Check sheet for the modelled part. Datum: model origin and axes. Units: mm. Coordinates: 2 decimals unless noted, no trailing zeros. Order: outer loops, then holes, each group sorted by start corner. A loop starts at its lowest first (then second) coordinate and runs counter-clockwise, first axis right, second up. Notation, with made-up numbers: (80.25, 52) -> (118.25, 52) arc R28 ccw to (118.25, 87) -> close; hole circle Ø5 at (-10.5, 13). An arc over 180 degrees is marked (long way). Put each result on its own line as item: value. Start each with the question number.
```python
from build123d import *

# Parameters (mm, degrees)
F0_W     = 255
F0_H     = 50
F1_DEPTH = 5
F2_R     = 3
F3_DEPTH = 5.001


with BuildPart() as f1:
    # F0 (on Top) → F1 (new body)
    with BuildSketch(Plane.XY):
        Polygon((200, -727.5), (200, 727.5), (-55, 727.5), (-200, 727.5), (-200, -727.5), (-55, -727.5), align=None)
        with Locations((72.5, -752.5)):
            Rectangle(F0_W, F0_H)
        with Locations((72.5, 752.5)):
            Rectangle(F0_W, F0_H)
    extrude(amount=F1_DEPTH)

    # F2 (on face) → F3 (cut, through all)
    with BuildSketch(Plane.XY.offset(5)):
        with Locations((135, 0)):
            Circle(F2_R)
        with Locations((-127.5, -700.58465)):
            Circle(F2_R)
        with Locations((135, -700.58465)):
            Circle(F2_R)
        with Locations((135, -350.292325)):
            Circle(F2_R)
        with Locations((-127.5, 700.58465)):
            Circle(F2_R)
        with Locations((135, 700.58465)):
            Circle(F2_R)
        with Locations((135, 350.292325)):
            Circle(F2_R)
    extrude(amount=-F3_DEPTH, mode=Mode.SUBTRACT)


solid = f1.part
```
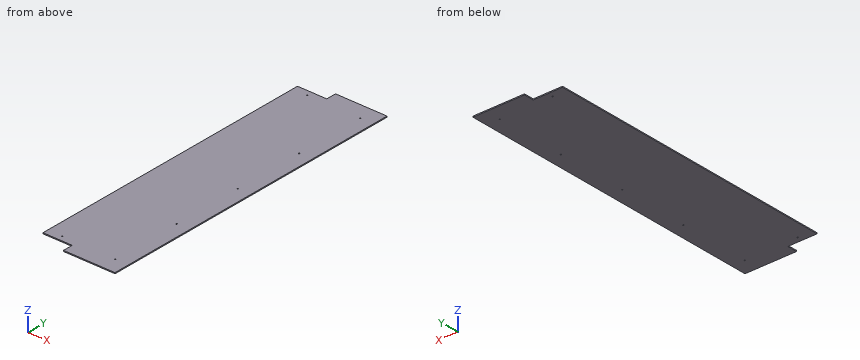
1) Scan lines: line 1 along Y through (x, z) = (135, 3.6); line 2 along Y through (x, z) = (-127.5, 1.1); line 3 along Y through (x, z) = (-72, 3.1). Record each from-to range of solid material in increasing order. Write a range as [from, to].
2) Gauge pin test, flat ends, axial feed: pin 1 (3 mm diameter, centred on x = -148.5, z = 2, fed in from -Y); pin 2 (3 mm diameter, centred on x = -123, z = 1, fed in from +Y); pin 3 (2.5 mm diameter, centred on y = -747, z = 2, fed in from -X). Record the tip position at first contact, or that the pin passes through.
3) Sectioned sample at A-A (x = -75.5). Record the boundary of the cut face in (y, z), plus the area to 4 significant figures.
Entries:
1. line 1: y = [-777.5, -703.58], [-697.58, -353.29], [-347.29, -3], [3, 347.29], [353.29, 697.58], [703.58, 777.5]
1. line 2: y = [-727.5, -703.58], [-697.58, 697.58], [703.58, 727.5]
1. line 3: y = [-727.5, 727.5]
2. pin 1: stops at y = -727.5
2. pin 2: stops at y = 727.5
2. pin 3: stops at x = -55
3. outline: (-727.5, 0) -> (727.5, 0) -> (727.5, 5) -> (-727.5, 5) -> close
3. area: 7,275 mm2
